The listing builds one solid part. Answer for the finished solid, in the listing's coordinates (mm). A direction names the side the tool comes from. Give positions to 0.01 mm unless a question says otherwise; leave off trailing zeros. Write each loop counter-clockwise with the first axis right and the second up, starting at its lowest first coordinate (ties: lowest second). Pieces come first, ordered by that corner, then holes. Notation, with made-up numbers: M -19.75,-4 L 23.25,-4 A23 cw 23.25,23 Z; hole C -10.5,-39.75 d2. An arc over 180 degrees is marked long. Return JSON: item names as keys, results as strings.
Autodesk Inventor part; units mm, degrees
ref_plane "YZ Plane" through (0, 0, 0) normal (1, 0, 0) x (0, 1, 0)
ref_plane "XZ Plane" through (0, 0, 0) normal (0, 1, 0) x (-1, 0, 0)
ref_plane "XY Plane" through (0, 0, 0) normal (0, 0, 1) x (1, 0, 0)
sketch "スケッチ1" plane through (0, 0, 0) normal (0, 1, 0) x (-1, 0, 0)
  line L0 (0, 0) -> (21, 0)
  line L1 (21, 0) -> (21, -75)
  line L2 (21, -75) -> (0, -75)
  line L3 (0, -75) -> (0, 0)
  dimension "d0" = 21
  dimension "d3" = 75
extrude "押し出し1" add sketch "スケッチ1" along normal blind 3
sketch "スケッチ2" plane through (0, 3, 0) normal (0, 1, 0) x (1, 0, 0)
  line L0 (-21, 0) -> (0, 0)
  line L1 (0, 75) -> (-21, 75)
  line L2 (-21, 75) -> (-21, 0)
  point P0 (-10.5, 10.65)
  point P1 (-10.5, 64.35)
  dimension "d4" = 53.7
  dimension "d5" = 10.65
  dimension "d7" = 10.5
hole "穴1" at (-10.5, 3, -10.65) at (-10.5, 3, -64.35) direction (0, -1, 0) diameter 3.2 end through all
sketch "スケッチ3" plane through (0, 3, 0) normal (0, 1, 0) x (1, 0, 0)
  line L0 (0, 75) -> (-21, 75)
  line L1 (-21, 0) -> (0, 0)
  line L2 (-21, 75) -> (0, 75)
  line L3 (0, 75) -> (0, 0)
  line L4 (0, 0) -> (-21, 0)
  line L5 (-21, 0) -> (-21, 75)
  line L6 (-18, 72) -> (-3, 72)
  line L7 (-3, 72) -> (-3, 3)
  line L8 (-3, 3) -> (-18, 3)
  line L9 (-18, 3) -> (-18, 72)
  dimension "d15" = 3
  dimension "d16" = 3
  dimension "d17" = 3
  dimension "d18" = 3
extrude "押し出し2" add sketch "スケッチ3" along normal blind 7.5
sketch "スケッチ4" plane through (0, 10.5, 0) normal (0, 1, 0) x (1, 0, 0)
  line L0 (0, 75) -> (-21, 75)
  line L1 (0, 0) -> (0, 75)
  line L2 (-21, 75) -> (0, 75)
  line L3 (0, 75) -> (0, 72)
  line L4 (0, 72) -> (-21, 72)
  line L5 (-21, 72) -> (-21, 75)
  line L6 (-21, 75) -> (-21, 0)
  line L7 (-21, 0) -> (0, 0)
  line L8 (0, 0) -> (0, 3)
  line L9 (0, 3) -> (-21, 3)
  line L10 (-21, 3) -> (-21, 0)
  dimension "d21" = 3
  dimension "d22" = 3
extrude "押し出し3" add sketch "スケッチ4" along normal blind 10.5 contours L1 L4 L5 L0 | L1 L7 L6 L9
properties part number "batteryBox" material "ポリプロピレン"
Item 1: Which of the six approach directions +Z, -Z, +X, -X, +Y, -Y give full straight-line access (tool end or side, diameter ignored) to faces 1 (the flat face through (-10, 3, -37)), 2 (the flat face through (-11, 10, 0)), 3 (the flat face through (-2, 10.5, -38))?
Geometry results:
{"face 1": "+Y", "face 2": "+Z, +X, -X, +Y, -Y", "face 3": "+X, -X, +Y"}
Item 2: A cutting plane is placed at B-B, the plane x = -10.5. Write down the section's boundary in (y, z), plus the area to 3 significant figures.
Geometry results:
{"outline": "M 0,-75 L 21,-75 L 21,-72 L 3,-72 L 3,-65.95 L 0,-65.95 Z; M 0,-62.75 L 3,-62.75 L 3,-12.25 L 0,-12.25 Z; M 0,-9.05 L 3,-9.05 L 3,-3 L 21,-3 L 21,0 L 0,0 Z", "area": "314 mm2"}
Item 3: Given pin 1 Ø3 at (y, z) = (9.5, -50) entering from +X; pin 2 Ø5 at (x, z) = (-11.5, -52.5) entering from +Y; pin 3 Ø2.5 at (x, z) = (-19.5, -22) entering from +Y; pin 4 Ø1 at (y, z) = (12.5, -21) entering from +X (3 decimals), each flat-ended and moving along its own axis, determine where each tip first touches the part or whether it passes through.
Geometry results:
{"pin 1": "stops at x = 0", "pin 2": "stops at y = 3", "pin 3": "stops at y = 10.5", "pin 4": "passes through"}
Item 4: A cutting plane is placed at A-A, the plane z = -10.65. Write down the section's boundary in (x, y), plus the area to 3 significant figures.
Geometry results:
{"outline": "M -21,0 L -12.1,0 L -12.1,3 L -18,3 L -18,10.5 L -21,10.5 Z; M -8.9,0 L 0,0 L 0,10.5 L -3,10.5 L -3,3 L -8.9,3 Z", "area": "98.4 mm2"}
Item 5: A cutting plane is placed at C-C, the plane y = 17. Write down the section's boundary in (x, z).
Geometry results:
{"outline": "M -21,-75 L 0,-75 L 0,-72 L -21,-72 Z; M -21,-3 L 0,-3 L 0,0 L -21,0 Z"}
Item 6: Determine the mould class of faces 4 (the flat face through (-20, 10.5, -38)), 5 (the flat face through (-10, 12, -72)), 6 (the flat face through (0, 6, -38)) for opening direction X: +X half, -X half, draft (parallel to the pull), parting line (faces both ways), or undercut.
Geometry results:
{"face 4": "draft", "face 5": "undercut", "face 6": "+X half"}
Item 7: Find the intervals of material crossed by line 1 (Z direction, x = -10.5, y = 1.1); line 2 (X direction, y = 10, z = -39); line 3 (Z direction, x = -6.5, y = 12.25), in increasing order.
Geometry results:
{"line 1": "z = -75 to -65.95, -62.75 to -12.25, -9.05 to 0", "line 2": "x = -21 to -18, -3 to 0", "line 3": "z = -75 to -72, -3 to 0"}
Item 8: A cutting plane is placed at D-D, the plane y = 7.5. Write down the section's boundary in (x, z).
Geometry results:
{"outline": "M -21,-75 L 0,-75 L 0,0 L -21,0 Z; hole M -18,-72 L -3,-72 L -3,-3 L -18,-3 Z"}
